Design review of the part built by this model. Coordinates are the model's own, in mm. A direction names the side the tool comes from. Give positions to 0.01 mm unless a question says otherwise; leave off trailing zeros. Write each loop counter-clockwise with the first axis right and the second up, starting at its lowest first coordinate (ties: lowest second). Pieces come first, ordered by that corner, then holes. Notation, with made-up numbers: M 46,64 L 53,64 A21 cw 53,91 Z; hole C -15.5,50.5 d6. An arc over 180 degrees is marked long. Answer in a Markdown table with one row per item.
```python
from build123d import *

# Parameters (mm, degrees)
BOSS_EXTRUDE1_DEPTH   = 6
BOSS_EXTRUDE1_2_DEPTH = 6
SKETCH1_3_R           = 10.5
SKETCH1_3_R_2         = 4.4
BOSS_EXTRUDE2_DEPTH   = 2
SKETCH2_R             = 8.575
BOSS_EXTRUDE3_DEPTH   = 4
SKETCH3_R             = 3
BOSS_EXTRUDE4_DEPTH   = 5
BOSS_EXTRUDE5_START   = -6
BOSS_EXTRUDE5_DEPTH   = 6
CUT_EXTRUDE1_REACH    = 31.079
SKETCH5_R             = 1.5
FILLET1_R             = 2
FILLET2_R             = 0.6


with BuildPart() as part:
    # Sketch1 → Boss-Extrude1 (new body)
    with BuildSketch(Plane(origin=(0, 0, 0), x_dir=(1, 0, 0), z_dir=(0, 1, 0))):
        with BuildLine():
            Line((-7.5, 13.5), (-7.5, 7.348469228))
            ThreePointArc((-7.5, 7.348469228), (0, 10.5), (7.5, 7.348469228))
            Line((7.5, 7.348469228), (7.5, 13.5))
            Line((7.5, 13.5), (-7.5, 13.5))
        make_face()
    extrude(amount=BOSS_EXTRUDE1_DEPTH)



with BuildPart() as body_2:
    # Sketch1 → Boss-Extrude1 2 (new body)
    with BuildSketch(Plane(origin=(0, 0, 0), x_dir=(1, 0, 0), z_dir=(0, 1, 0))):
        with BuildLine():
            ThreePointArc((7.5, -7.348469228), (0, -10.5), (-7.5, -7.348469228))
            Line((-7.5, -7.348469228), (-7.5, -13.5))
            Line((-7.5, -13.5), (7.5, -13.5))
            Line((7.5, -13.5), (7.5, -7.348469228))
        make_face()
    extrude(amount=BOSS_EXTRUDE1_2_DEPTH)


with BuildPart() as part_1:
    add(part.part)

    add(body_2.part)  # Boss-Extrude2 merges body 2
    # Sketch1<3> → Boss-Extrude2 (add)
    with BuildSketch(Plane(origin=(0, 0, 0), x_dir=(1, 0, 0), z_dir=(0, 1, 0))):
        Circle(SKETCH1_3_R)
        with Locations(Location((0, 0, 0), (0, 0, 270))):
            Circle(SKETCH1_3_R_2, mode=Mode.SUBTRACT)
    extrude(amount=BOSS_EXTRUDE2_DEPTH)

    # Sketch2 → Boss-Extrude3 (add)
    with BuildSketch(Plane(origin=(0, 2, 0), x_dir=(1, 0, 0), z_dir=(0, 1, 0))):
        with BuildLine():
            ThreePointArc((7.5, 7.348469228), (0, 10.5), (-7.5, 7.348469228))
            ThreePointArc((-7.5, 7.348469228), (-10.5, 0), (-7.5, -7.348469228))
            ThreePointArc((-7.5, -7.348469228), (0, -10.5), (7.5, -7.348469228))
            ThreePointArc((7.5, -7.348469228), (10.5, 0), (7.5, 7.348469228))
        make_face()
        with Locations(Location((0, 0, 0), (0, 0, 270))):
            Circle(SKETCH2_R, mode=Mode.SUBTRACT)
    extrude(amount=BOSS_EXTRUDE3_DEPTH)

    # Sketch3 → Boss-Extrude4 (add)
    with BuildSketch(Plane(origin=(0, 0, -13.5), x_dir=(-1, 0, 0), z_dir=(0, 0, -1))):
        with Locations(Location((0, 3, 0), (0, 0, 270))):
            Circle(SKETCH3_R)
    boss_extrude4 = extrude(amount=BOSS_EXTRUDE4_DEPTH)

    # Mirror1: Boss-Extrude4 across plane
    add(boss_extrude4.mirror(Plane.XY))

    # Sketch4 → Boss-Extrude5 (add)
    with BuildSketch(Plane(origin=(0, 6, 0), x_dir=(1, 0, 0), z_dir=(0, 1, 0)).offset(BOSS_EXTRUDE5_START)):
        with BuildLine():
            Line((10.198039027, -2.5), (19.198039027, -2.5))
            Line((19.198039027, -2.5), (19.198039027, 2.5))
            Line((19.198039027, 2.5), (10.198039027, 2.5))
            ThreePointArc((10.198039027, 2.5), (10.5, 0), (10.198039027, -2.5))
        make_face()
    extrude(amount=BOSS_EXTRUDE5_DEPTH)

    # Sketch5 → Cut-Extrude1 (cut, up to next)
    with BuildSketch(Plane(origin=(0, 0, -2.5), x_dir=(-1, 0, 0), z_dir=(0, 0, -1)), mode=Mode.PRIVATE) as cut_extrude1_sk1:
        with Locations((-16.198039027, 3)):
            Circle(SKETCH5_R)
    cut_extrude1_tool1 = extrude(cut_extrude1_sk1.sketch, amount=-CUT_EXTRUDE1_REACH, mode=Mode.PRIVATE) & part_1.part
    add(cut_extrude1_tool1.solids().sort_by_distance((16.198039, 3, -2.5))[0], mode=Mode.SUBTRACT)

    # Fillet1
    fillet1_edges = [part_1.edges().sort_by_distance(p)[0] for p in [
        (7.5, 3, 7.348469228),
        (-7.5, 3, 13.5),
        (7.5, 3, 13.5),
        (19.198039027, 6, 0),
        (19.198039027, 0, 0),
        (-7.5, 3, -7.348469228),
        (-7.5, 3, -13.5),
        (7.5, 3, -13.5),
        (7.5, 3, -7.348469228),
    ]]
    fillet(fillet1_edges, radius=FILLET1_R)

    # Fillet2
    fillet2_edges = [part_1.edges().sort_by_distance(p)[0] for p in [
        (10.198039027, 3, 2.5),
        (10.198039027, 3, -2.5),
    ]]
    fillet(fillet2_edges, radius=FILLET2_R)


with BuildPart() as body_2_2:
    # Mirror3: mirrored copy
    add(part_1.part.mirror(Plane.ZX.offset(16)))


solid = body_2_2.part
```
1) Add section A-A (y = 29). Count the separate pieces of the cut face and the enclosed holes in it, and give its area (3 significant figures).
Geometry says:
| item | result |
|---|---|
| separate pieces | 2 |
| enclosed holes | 1 |
| area | 321 mm^2 |
2) Insertion check: P1, Ø3, axis at x = 14, y = 28, coming from the +Z side; P2, Ø2, axis at y = 29.5, z = 10, coming from the -X side; P3, Ø2.5, axis at y = 30, z = 9, coming from the +X side. Each pin has a flat end and moves straight along its axis. Give the tip position at first contact, or say it passes through.
Geometry says:
| item | result |
|---|---|
| P1 | z = 2.5 |
| P2 | x = -7.5 |
| P3 | x = 7.54 |
3) Add section B-B (z = 0). Write out the cut boundary in (x, y) (3 decimals), and give its area (3 significant figures).
Geometry says:
| item | result |
|---|---|
| outline | M -10.5,26 L -8.575,26 L -8.575,30 L -4.4,30 L -4.4,32 L -10.5,32 Z; M 4.4,30 L 8.575,30 L 8.575,26 L 17.198,26 A2 ccw 19.198,28 L 19.198,30 A2 ccw 17.198,32 L 4.4,32 Z; hole C 16.198,29 d3 |
| area | 83.2 mm^2 |
4) Add section C-C (z = -16). Write out the cut boundary in (x, y), and give its area (3 significant figures).
Geometry says:
| item | result |
|---|---|
| outline | C 0,29 d6 |
| area | 28.3 mm^2 |
5) The part is to be moulded in two halves that separate along X. For faces 1 (the face through (7.5, 29, -10)), 2 (the face through (4, 29, 13.5)), 3 (the face through (4, 30, 4)), say which applies: released by +X, released by -X, zero draft, split by the parting line, or undercut.
Geometry says:
| item | result |
|---|---|
| face 1 | released by +X |
| face 2 | zero draft |
| face 3 | undercut |
6) To check wall thickness, follow probe 1 along X at (y, z) = (29.05, 0) (3 decimals); probe 2 along Y at (x, z) = (-5, 6); probe 3 along X at (y, z) = (31.5, 9). State the ranges of each line that lie inside material, in increasing order. Write a range as [from, to].
Geometry says:
| item | result |
|---|---|
| probe 1 | [-10.5, -8.575], [8.575, 14.699], [17.697, 19.198] |
| probe 2 | [30, 32] |
| probe 3 | [-7.5, 7.5] |
7) For faces 4 (the face through (14, 29, -2.5)), 5 (the face through (0, 26, 16)), 6 (the face through (2.576, 28.028, 8.179)), 7 (the face through (0, 26, -16)), 8 (the face through (-7.5, 29, -10)), list the 3-axis set-ups (+Z, -Z, +X, -X, +Y, -Y) from which the entire face can be reached by the end or side of a thin tool; tool diameter is ignored.
Geometry says:
| item | result |
|---|---|
| face 4 | -Z, +X, +Y, -Y |
| face 5 | +Z |
| face 6 | -Y |
| face 7 | -Z |
| face 8 | -Z, -X, +Y, -Y |
